For this review, take the finished solid that the model builds, in its own axes (mm). Face numbers are marked on the shaded views. A direction names the side the tool comes from. Give positions to 0.01 mm unless a question says otherwise; leave off trailing zeros. Order: outer loops, then holes, each group sorted by start corner. A loop starts at its lowest first (then second) coordinate and runs counter-clockwise, first axis right, second up. Notation, with made-up numbers: (28, -21.75) - (44, -21.75) arc R32 cw to (44, 4.25) - close; hole circle Ø5 at (8.25, 17.25). An arc over 180 degrees is marked (long way). Answer as a JSON object with one key per item and string values. Group by question number.
from build123d import *

# Parameters (mm, degrees)
SKIZZE1_W                       = 70
SKIZZE1_H                       = 30
SKIZZE1_R                       = 4
SKIZZE1_R_2                     = 0.1
LINEAR_AUSTRAGEN1_DEPTH         = 3
F_1_0_1_DIAMETER_HOLE1_D        = 1
F_2_0_2_DIAMETER_HOLE1_D        = 2
SKIZZE7_R                       = 8.5
SCHNITT_LINEAR_AUSTRAGEN1_DEPTH = 1
SKIZZE8_OUTSIDE_W               = 87.244
SKIZZE8_OUTSIDE_H               = 47.244
SCHNITT_LINEAR_AUSTRAGEN2_DEPTH = 4
SCHNITT_LINEAR_AUSTRAGEN3_DEPTH = 1.2


with BuildPart() as part:
    # Skizze1 → Linear austragen1 (new body)
    with BuildSketch(Plane.XY):
        with Locations((20, 0)):
            Rectangle(SKIZZE1_W, SKIZZE1_H)
        Circle(SKIZZE1_R, mode=Mode.SUBTRACT)
        with Locations((40, 0)):
            Circle(SKIZZE1_R_2, mode=Mode.SUBTRACT)
    extrude(amount=LINEAR_AUSTRAGEN1_DEPTH)

    # 1.0 _1_ Diameter Hole1 (through all)
    with Locations(Plane(origin=(0, 0, 0), x_dir=(-1, 0, 0), z_dir=(0, 0, -1))):
        with Locations((6.5, 0), (-6.5, 0)):
            Hole(F_1_0_1_DIAMETER_HOLE1_D / 2)

    # 2.0 _2_ Diameter Hole1 (through all)
    with Locations(Plane(origin=(0, 0, 0), x_dir=(1, 0, 0), z_dir=(0, 0, -1))):
        with Locations((12.5, 3)):
            Hole(F_2_0_2_DIAMETER_HOLE1_D / 2)

    # Skizze7 → Schnitt-Linear austragen1 (cut)
    with BuildSketch(Plane.XY):
        Circle(SKIZZE7_R)
    extrude(amount=SCHNITT_LINEAR_AUSTRAGEN1_DEPTH, mode=Mode.SUBTRACT)

    # Skizze8 outside → Schnitt-Linear austragen2 (cut, through all)
    with BuildSketch(Plane.XY):
        with Locations((20, 0)):
            Rectangle(SKIZZE8_OUTSIDE_W, SKIZZE8_OUTSIDE_H)
        with BuildLine():
            Line((-4.242640687, 6.5), (4.850693198, 6.5))
            ThreePointArc((4.850693198, 6.5), (5.911913676, 6.386083411), (6.924777907, 6.049524439))
            ThreePointArc((6.924777907, 6.049524439), (22.851496839, 1.777066749), (39.30182783, 2.917628424))
            ThreePointArc((39.30182783, 2.917628424), (43, 0), (39.30182783, -2.917628424))
            ThreePointArc((39.30182783, -2.917628424), (29.897933333, -1.594625688), (20.413511825, -2.073495804))
            ThreePointArc((20.413511825, -2.073495804), (17.039126957, -3.208684673), (14.276292568, -5.454096248))
            ThreePointArc((14.276292568, -5.454096248), (13.252539671, -6.226012541), (12, -6.5))
            Line((12, -6.5), (-4.242640687, -6.5))
            ThreePointArc((-4.242640687, -6.5), (-7.129392033, -5.582482905), (-8.956685895, -3.166666667))
            ThreePointArc((-8.956685895, -3.166666667), (-9.5, 0), (-8.956685895, 3.166666667))
            ThreePointArc((-8.956685895, 3.166666667), (-7.129392033, 5.582482905), (-4.242640687, 6.5))
        make_face(mode=Mode.SUBTRACT)
    extrude(amount=SCHNITT_LINEAR_AUSTRAGEN2_DEPTH, mode=Mode.SUBTRACT)

    # Skizze10 → Schnitt-Linear austragen3 (cut)
    with BuildSketch(Plane.XY):
        with BuildLine():
            ThreePointArc((9.699012563, -0.995818907), (9.689735111, 1.082373999), (9.240224203, 3.111391438))
            ThreePointArc((9.240224203, 3.111391438), (9.397134344, 3.759216075), (10.049282761, 3.89705654))
            ThreePointArc((10.049282761, 3.89705654), (23.054109204, 0.954513618), (36.376629725, 1.49720748))
            ThreePointArc((36.376629725, 1.49720748), (36.94164037, 1.30691696), (37.090043464, 0.729488148))
            ThreePointArc((37.090043464, 0.729488148), (37, 0), (37.090043464, -0.729488148))
            ThreePointArc((37.090043464, -0.729488148), (36.94164037, -1.30691696), (36.376629725, -1.49720748))
            ThreePointArc((36.376629725, -1.49720748), (28.345625064, -0.749320212), (20.297478014, -1.281955435))
            ThreePointArc((20.297478014, -1.281955435), (17.915226797, -1.915501516), (15.73868827, -3.072731627))
            ThreePointArc((15.73868827, -3.072731627), (15.136326342, -3.131711101), (14.766431088, -2.652653724))
            ThreePointArc((14.766431088, -2.652653724), (13.150598424, -0.801345638), (10.787531238, -1.47526722))
            ThreePointArc((10.787531238, -1.47526722), (10.068812364, -1.631628436), (9.699012563, -0.995818907))
        make_face()
    extrude(amount=SCHNITT_LINEAR_AUSTRAGEN3_DEPTH, mode=Mode.SUBTRACT)


with BuildPart() as body_2:
    # Mirror1: mirrored copy
    add(part.part.mirror(Plane(origin=(-15, -15, 3), x_dir=(1, 0, 0), z_dir=(0, 0, 1))))


solid = body_2.part
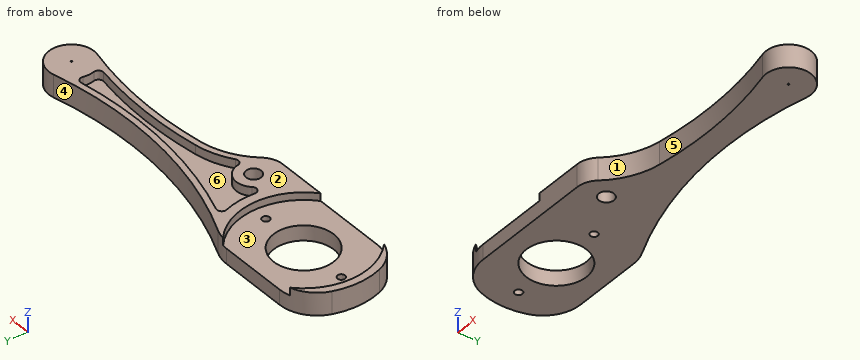
1) Consider section C-C (x = 30). Give the boundary of the cut face in (y, z).
2) For pin 1 (1.5 mm diameter, centred on y = -5, z = 5, fed in from +X) (3 decimals); pin 2 (1 mm diameter, centred on y = -1, z = 4, fed in from -X), all flat-tipped, find the tip position at first contact; note any pin that passes through.
3) Consider section A-A (x = 13). Give the boundary of the cut face in (y, z), plus the area to 3 significant figures.
4) Consider section D-D (x = 22). Give the boundary of the cut face in (y, z), plus the area to 3 significant figures.
5) Consider section B-B (z = 3.85). Give the boundary of the cut face in (x, y).
6) For line 1 (X direction, y = 0.25, z = 5.7); line 2 (Y direction, x = 0, z = 3.4); line 3 (Y direction, x = -3.5, z = 3.65), list the stretches that pass through material, from the lowest coordinate up.
7) Mouldability with a two-part tool opening along Y and no side actions: class the marked faces 4, 5 and 6 as released by +Y, released by -Y, zero draft, split by the parting line, or undercut.
8) For the marked faces 1, 2 and 3, list the 3-axis set-ups (+Z, -Z, +X, -X, +Y, -Y) from which the entire face can be reached by the end or side of a thin tool; tool diameter is ignored.
Result set:
{
 "1": {"outline": "(-1.6, 3) - (1.6, 3) - (1.6, 6) - (0.8, 6) - (0.8, 4.8) - (-0.8, 4.8) - (-0.8, 6) - (-1.6, 6) - close"},
 "2": {"pin 1": "stops at x = 15.505", "pin 2": "stops at x = -9.49"},
 "3": {"outline": "(-6.33, 3) - (-3.87, 3) - (-3.87, 6) - (-6.33, 6) - close; (-2.13, 3) - (3.74, 3) - (3.74, 6) - (2.91, 6) - (2.91, 4.8) - (-0.76, 4.8) - (-0.76, 6) - (-2.13, 6) - close", "area": "20.6 mm2"},
 "4": {"outline": "(-1.87, 3) - (1.87, 3) - (1.87, 6) - (1.06, 6) - (1.06, 4.8) - (-1.06, 4.8) - (-1.06, 6) - (-1.87, 6) - close", "area": "8.65 mm2"},
 "5": {"outline": "(-8.96, -3.17) arc R5 ccw to (-4.24, -6.5) - (12, -6.5) arc R3 ccw to (14.28, -5.45) arc R10 cw to (20.41, -2.07) arc R50 cw to (39.3, -2.92) arc R3 ccw (long way) to (39.3, 2.92) arc R50 cw to (6.92, 6.05) arc R5 ccw to (4.85, 6.5) - (-4.24, 6.5) arc R5 ccw to (-8.96, 3.17) arc R9.5 ccw to start; hole circle Ø1 at (-6.5, 0); hole circle Ø8 at (0, 0); hole circle Ø1 at (6.5, 0); hole circle Ø2 at (12.5, -3); hole circle Ø0.2 at (40, 0)"},
 "6": {"line 1": "x = -9.5 to -8.5, 8.5 to 9.75, 37.01 to 42.99", "line 2": "y = -6.5 to -4, 4 to 6.5", "line 3": "y = -6.5 to -1.94, 1.94 to 6.5"},
 "7": {"face 4": "released by +Y", "face 5": "released by -Y", "face 6": "undercut"},
 "8": {"face 1": "+Z, -Z, -Y", "face 2": "+Z, +X, -X, +Y, -Y", "face 3": "+Z"}
}
